Source: CAD feature listing. Evaluate the final solid. Frame: model axes, mm. Face numbers are marked on the shaded views. Round coordinates to 2 decimals unless told otherwise and drop trailing zeros. Order: outer loops, then holes, each group sorted by start corner. A loop starts at its lowest first (then second) coordinate and runs counter-clockwise, first axis right, second up. Notation, with made-up numbers: (-0.5, 3.5) -> (52.5, 3.5) arc R25 cw to (52.5, 39.5) -> close; hole circle Ø4 at (9, 37). An arc over 180 degrees is marked (long way). One line per item, written item: value. Start each with the question number.
1) Mould query, pull axis X, two halves, no side actions, for the marked faces 1, 2 and 3. Classes: pulls with the +X half, pulls with the -X half, needs draft (parallel to the pull), parting line crosses it, or undercut.
2) Section C-C (x = -2.5). Return the cut outline in (y, z), and give its area (3 significant figures).
3) Ray query, L1, parallel to X at y = -6, z = 5.5; L2, parallel to X at y = -3.5, z = 2.25; L3, parallel to X at y = 10.5, z = 10.75. Return the intervals inside material, ascending.
4) Pin query (flat end, axial travel): P1, Ø5, axis at x = -3.07, y = 9.02, coming from the -Z side; P2, Ø1.5, axis at x = -8, z = 9.5, coming from the +Y side; P3, Ø3, axis at y = 8, z = 11.5, coming from the +X side. Return the tip coordinate at first contact, or that it passes through.
5) Section B-B (x = -9.5). Return the cut outline in (y, z), and give its area (3 significant figures).
6) Section A-A (y = -2.5). Return the cut outline in (x, z).
7) Section D-D (z = 4). State how many separate pieces and enclosed holes the cut face has, and give its area (3 significant figures).
```python
from build123d import *

# Parameters (mm, degrees)
SKETCH1_R           = 12.7
SKETCH1_R_2         = 3.96875
BOSS_EXTRUDE1_DEPTH = 12.7
CUT_EXTRUDE1_DEPTH  = 22.997045256
CIRPATTERN1_COUNT   = 12


with BuildPart() as part:
    # Sketch1 → Boss-Extrude1 (new body)
    with BuildSketch(Plane.XY):
        Circle(SKETCH1_R)
        Circle(SKETCH1_R_2, mode=Mode.SUBTRACT)
    extrude(amount=BOSS_EXTRUDE1_DEPTH)

    # Sketch2 → Cut-Extrude1 (cut, through all)
    with BuildSketch(Plane.XY.offset(12.7)):
        with BuildLine():
            Line((-4.354775644, 7.61249898), (-1.77319664, 5.248090699))
            Line((-1.77319664, 5.248090699), (-1.260387004, 8.416402273))
            Line((-1.260387004, 8.416402273), (-1.163123324, 9.017330218))
            ThreePointArc((-1.163123324, 9.017330218), (-3.83557115, 10.7609038), (-4.354775644, 7.61249898))
        make_face()
    cut_extrude1 = extrude(amount=-CUT_EXTRUDE1_DEPTH, mode=Mode.SUBTRACT)

    # CirPattern1: Cut-Extrude1 ×12 about axis
    cirpattern1_axis = Axis((0, 0, 0), (0, 0, 1))
    for i in range(1, CIRPATTERN1_COUNT):
        add(cut_extrude1.rotate(cirpattern1_axis, i * 360 / CIRPATTERN1_COUNT), mode=Mode.SUBTRACT)


solid = part.part
```
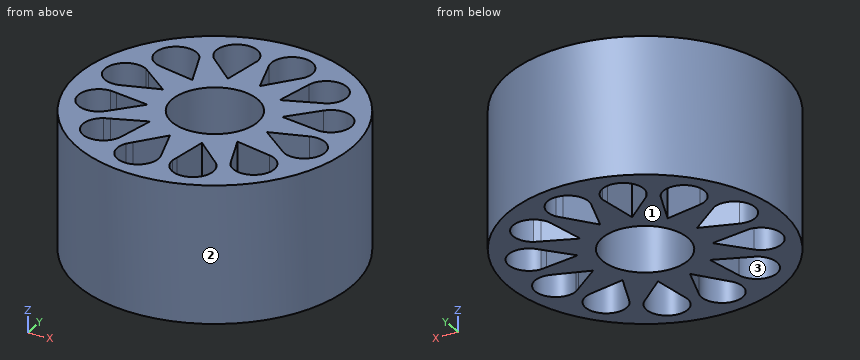
Findings:
1. face 1: needs draft
1. face 2: parting line crosses it
1. face 3: undercut
2. outline: (-12.45, 0) -> (-11.13, 0) -> (-11.13, 12.7) -> (-12.45, 12.7) -> close; (-7.16, 0) -> (-3.08, 0) -> (-3.08, 12.7) -> (-7.16, 12.7) -> close; (3.08, 0) -> (5.91, 0) -> (5.91, 12.7) -> (3.08, 12.7) -> close; (10.84, 0) -> (12.45, 0) -> (12.45, 12.7) -> (10.84, 12.7) -> close
2. area: 125 mm2
3. L1: -11.19 to -7.78, -4.07 to -1.55, -0.91 to 1.65, 2.59 to 5.05, 9.05 to 11.19
3. L2: -12.21 to -10.87, -6.83 to -1.87, 1.87 to 8.39, 10.3 to 12.21
3. L3: -7.14 to -4.26, -1.87 to 0.34, 3.37 to 7.14
4. P1: z = 0
4. P2: y = 10.43
4. P3: x = 10.91
5. outline: (-8.43, 0) -> (-4.91, 0) -> (-4.91, 12.7) -> (-8.43, 12.7) -> close; (-1.23, 0) -> (-0.05, 0) -> (-0.05, 12.7) -> (-1.23, 12.7) -> close; (3.75, 0) -> (8.43, 0) -> (8.43, 12.7) -> (3.75, 12.7) -> close
5. area: 119 mm2
6. outline: (-12.45, 0) -> (-10.84, 0) -> (-10.84, 12.7) -> (-12.45, 12.7) -> close; (-5.91, 0) -> (-3.08, 0) -> (-3.08, 12.7) -> (-5.91, 12.7) -> close; (3.08, 0) -> (7.16, 0) -> (7.16, 12.7) -> (3.08, 12.7) -> close; (11.13, 0) -> (12.45, 0) -> (12.45, 12.7) -> (11.13, 12.7) -> close
7. separate pieces: 1
7. enclosed holes: 13
7. area: 288 mm2
